Geometry: final body of the model. Coordinates: model frame, mm. Face numbers are marked on the shaded views. A direction names the side the tool comes from. Give positions to 0.01 mm unless a question says otherwise; leave off trailing zeros. Loops run counter-clockwise (first coordinate to the right, second up) from the corner with the lowest first, then second, coordinate; pieces in that order, holes last.
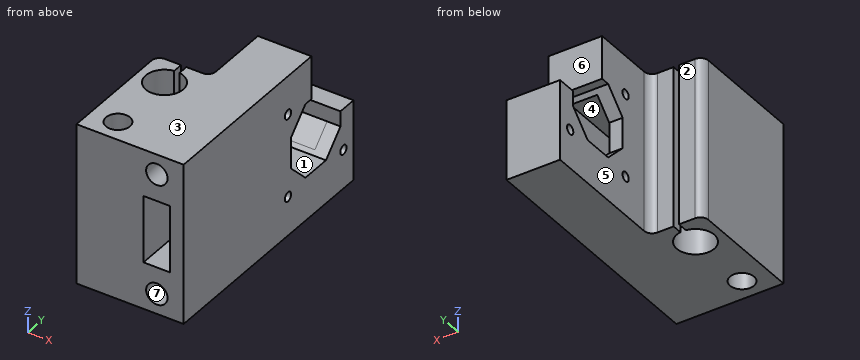
```python
from build123d import *

# Parameters (mm, degrees)
SKETCH060_W              = 45
SKETCH060_H              = 20
SKETCH060_R              = 4.5
SKETCH060_R_2            = 7
PAD033_DEPTH             = 60
SKETCH061_W              = 4
SKETCH061_H              = 2
POCKET031_DEPTH          = 60.001
POCKET031_FACE6_W        = 45
POCKET031_FACE6_H        = 60
PAD034_DEPTH             = 20
SKETCH062_W              = 10
SKETCH062_H              = 25
POCKET032_DEPTH          = 47
SKETCH063_R              = 4
POCKET033_DEPTH          = 20
POCKET033_FACE21_W       = 20
POCKET033_FACE21_H       = 60
POCKET033_FACE21_W_2     = 10
POCKET033_FACE21_H_2     = 25
PAD035_DEPTH             = 50
FILLET004_R              = 3
FILLET005_R              = 3
SKETCH064_R              = 1.75
POCKET034_DEPTH          = 20.001
SKETCH065_W              = 23.5
SKETCH065_H              = 30
POCKET035_DEPTH          = 20.001
POCKET035_FACE41_W       = 10
POCKET035_FACE41_H       = 14.1015555269
PAD036_DEPTH             = 12.5
POCKET036_DEPTH          = 35.001
BODY019_PLACEMENT_ANGLE  = 180
CLONE047_PLACEMENT_ANGLE = 90


with BuildPart() as part:
    # Sketch060 → Pad033 (new body)
    with BuildSketch(Plane.XY):
        Rectangle(SKETCH060_W, SKETCH060_H)
        with Locations((-14.26955, 0)):
            Circle(SKETCH060_R, mode=Mode.SUBTRACT)
        with Locations((11.73045, 0)):
            Circle(SKETCH060_R_2, mode=Mode.SUBTRACT)
    extrude(amount=PAD033_DEPTH)

    # Sketch061 (on Face8 of Pad033) → Pocket031 (cut, through all)
    with BuildSketch(Plane.XY.offset(60)):
        with Locations((20.51, 0)):
            Rectangle(SKETCH061_W, SKETCH061_H)
    extrude(amount=-POCKET031_DEPTH, mode=Mode.SUBTRACT)

    # Pocket031 Face6 → Pad034 (add)
    with BuildSketch(Plane(origin=(0, -10, 30), x_dir=(-1, 0, 0), z_dir=(0, -1, 0))):
        Rectangle(POCKET031_FACE6_W, POCKET031_FACE6_H)
    extrude(amount=PAD034_DEPTH)

    # Sketch062 (on Face6 of Pad034) → Pocket032 (cut)
    with BuildSketch(Plane(origin=(-22.5, 0, 0), x_dir=(0, -1, 0), z_dir=(-1, 0, 0))):
        with Locations((20, 30)):
            Rectangle(SKETCH062_W, SKETCH062_H)
    extrude(amount=-POCKET032_DEPTH, mode=Mode.SUBTRACT)

    # Sketch063 (on Face6 of Pocket032) → Pocket033 (cut)
    with BuildSketch(Plane(origin=(-22.5, 0, 0), x_dir=(0, -1, 0), z_dir=(-1, 0, 0))):
        with Locations((20, 52.5)):
            Circle(SKETCH063_R)
        with Locations((20, 7.5)):
            Circle(SKETCH063_R)
    extrude(amount=-POCKET033_DEPTH, mode=Mode.SUBTRACT)

    # Pocket033 Face21 → Pad035 (add)
    with BuildSketch(Plane(origin=(22.5, -20, 30), x_dir=(0, -1, 0), z_dir=(1, 0, 0))):
        Rectangle(POCKET033_FACE21_W, POCKET033_FACE21_H)
        Rectangle(POCKET033_FACE21_W_2, POCKET033_FACE21_H_2, mode=Mode.SUBTRACT)
    extrude(amount=PAD035_DEPTH)

    # Fillet004
    fillet004_edges = [part.edges().sort_by_distance(p)[0] for p in [
        (22.5, -10, 30),
    ]]
    fillet(fillet004_edges, radius=FILLET004_R)

    # Fillet005
    fillet005_edges = [part.edges().sort_by_distance(p)[0] for p in [
        (22.5, 10, 30),
    ]]
    fillet(fillet005_edges, radius=FILLET005_R)

    # Sketch064 (on Face16 of Fillet005) → Pocket034 (cut, through all)
    with BuildSketch(Plane(origin=(0, -10, 0), x_dir=(-1, 0, 0), z_dir=(0, 1, 0))):
        with Locations((-35.85, 45.55)):
            Circle(SKETCH064_R)
        with Locations((-66.85, 45.55)):
            Circle(SKETCH064_R)
        with Locations((-66.85, 14.55)):
            Circle(SKETCH064_R)
        with Locations((-35.85, 14.55)):
            Circle(SKETCH064_R)
        Polygon((-37.4918070123, 35.7902514855), (-45.6097485145, 43.9081929877), (-57.0902514855, 43.9081929877), (-65.2081929877, 35.7902514855), (-65.2081929877, 24.3097485145), (-57.0902514855, 16.1918070123), (-45.6097485145, 16.1918070123), (-37.4918070123, 24.3097485145), align=None)
    extrude(amount=-POCKET034_DEPTH, mode=Mode.SUBTRACT)

    # Sketch065 (on Face16 of Pocket034) → Pocket035 (cut, through all)
    with BuildSketch(Plane(origin=(0, -10, 0), x_dir=(-1, 0, 0), z_dir=(0, 1, 0))):
        with Locations((-60.75, 45)):
            Rectangle(SKETCH065_W, SKETCH065_H)
    extrude(amount=-POCKET035_DEPTH, mode=Mode.SUBTRACT)

    # Pocket035 Face41 → Pad036 (add)
    with BuildSketch(Plane(origin=(65.4492222366, -20, 17.5), x_dir=(0, 1, 0), z_dir=(0, 0, 1))):
        Rectangle(POCKET035_FACE41_W, POCKET035_FACE41_H)
    extrude(amount=PAD036_DEPTH)

    # Pad036 Face50 → Pocket036 (cut, through all)
    with BuildSketch(Plane(origin=(61.3784329533, -25, 25.2399942401), x_dir=(-1, 0, 0), z_dir=(0, -1, 0))):
        Polygon((2.9799884801, 7.7399942401), (-3.8297600344, 0.9302457255), (-3.8297600344, -4.7600057599), (2.9799884801, -4.7600057599), align=None)
    extrude(amount=-POCKET036_DEPTH, mode=Mode.SUBTRACT)


with BuildPart() as part_1:
    # Body019 placement: moved
    add(part.part.moved(Location((-73, 0, 0))).rotate(Axis((-73, 0, 0), (0, 0, 1)), BODY019_PLACEMENT_ANGLE))


with BuildPart() as part_2:
    # Clone047 placement: moved
    add(part_1.part.moved(Location((-310, -84, 92))).rotate(Axis((-310, -84, 92), (0, 0, -1)), CLONE047_PLACEMENT_ANGLE))


solid = part_2.part
```
Q1. Section query B-B, the plane x = -290. Return loops of the section in (y, z), and give its area (3 significant figures).
Q2. Material intervals for probe 1 along Y at (x, z) = (-287.25, 106.55); probe 2 along Z at (x, y) = (-290, -26); probe 3 along Y at (x, z) = (-288.5, 107), sorted ascending.
Q3. Pin query (flat end, axial travel): pin 1 Ø2.5 at (x, z) = (-297, 125) entering from +Y; pin 2 Ø3 at (y, z) = (13.5, 142) entering from -X; pin 3 Ø14 at (y, z) = (31, 127) entering from -X. Return the tip coordinate at first contact, or that it passes through.
Q4. Section query D-D, the plane z = 111.5. Return loops of the section in (x, y).
Q5. Section query A-A, the plane z = 137.55. Return loops of the section in (x, y), and give its area (3 significant figures).
Q6. Reachability of the marked faces 4, 5, 6 and 7 from +Z, -Z, +X, -X, +Y, -Y: full face, straight path, thin tool, end or side. Return the list, or none.
Q7. Mould query, pull axis Y, two halves, no side actions, for the marked faces 1, 2 and 3. Classes: +Y half, -Y half, draft (parallel to the pull), parting line (faces both ways), or undercut.
Q8. Section query C-C, the plane y = 24.85. Return loops of the section in (x, z).
Resolved:
1. outline: (-33.5, 92) - (61.5, 92) - (61.5, 122) - (54.21, 122) - (54.21, 116.31) - (46.09, 108.19) - (34.61, 108.19) - (33.3, 109.5) - (-33.5, 109.5) - (-33.5, 103.5) - (-13.5, 103.5) - (-13.5, 95.5) - (-33.5, 95.5) - close; (-33.5, 134.5) - (33.2, 134.5) - (34.61, 135.91) - (38, 135.91) - (38, 152) - (-33.5, 152) - (-33.5, 148.5) - (-13.5, 148.5) - (-13.5, 140.5) - (-33.5, 140.5) - close; hole circle Ø3.5 at (24.85, 106.55); hole circle Ø3.5 at (24.85, 137.55); hole circle Ø3.5 at (55.85, 106.55)
1. area: 2,660 mm2
2. probe 1: y = -33.5 to 23.1, 26.6 to 54.1, 57.6 to 61.5
2. probe 2: z = 92 to 95.5, 103.5 to 109.5, 134.5 to 140.5, 148.5 to 152
2. probe 3: y = -33.5 to 23.16, 26.54 to 54.16, 57.54 to 61.5
3. pin 1: stops at y = 26.49
3. pin 2: stops at x = -301.34
3. pin 3: stops at x = -300
4. outline: (-320, -33.5) - (-295, -33.5) - (-295, 31.3) - (-300, 31.3) - (-300, 14.5) arc R3 cw to (-303, 11.5) - (-309, 11.5) - (-309, 7.66) arc R7 cw (long way) to (-311, 7.66) - (-311, 11.5) - (-317, 11.5) arc R3 ccw to (-320, 8.5) - close; (-300, 49.4) - (-280, 49.4) - (-280, 61.5) - (-300, 61.5) - close; (-285, -33.5) - (-280, -33.5) - (-280, 31.3) - (-285, 31.3) - close; hole circle Ø9 at (-310, -25.27)
5. outline: (-320, -33.5) - (-280, -33.5) - (-280, 23.1) - (-300, 23.1) - (-300, 14.5) arc R3 cw to (-303, 11.5) - (-309, 11.5) - (-309, 7.66) arc R7 cw (long way) to (-311, 7.66) - (-311, 11.5) - (-317, 11.5) arc R3 ccw to (-320, 8.5) - close; (-300, 26.6) - (-280, 26.6) - (-280, 38) - (-300, 38) - close; hole circle Ø9 at (-310, -25.27)
5. area: 2,030 mm2
6. face 4: +Y, -Y
6. face 5: +Z, -Z, -X, +Y
6. face 6: +Z, +X, -X, +Y
6. face 7: -Y
7. face 1: undercut
7. face 2: +Y half
7. face 3: draft
8. outline: (-300, 92) - (-280, 92) - (-280, 104.8) - (-300, 104.8) - close; (-300, 108.3) - (-280, 108.3) - (-280, 135.8) - (-300, 135.8) - close; (-300, 139.3) - (-280, 139.3) - (-280, 152) - (-300, 152) - close; hole (-295, 109.5) - (-285, 109.5) - (-285, 134.5) - (-295, 134.5) - close
